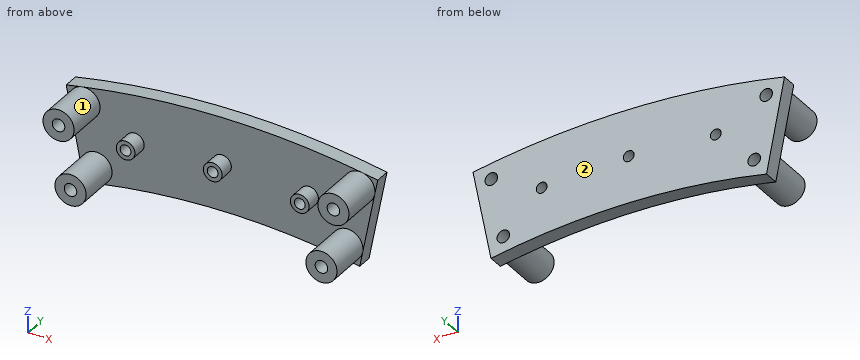
from build123d import *

# Parameters (mm, degrees)
F1_DEPTH = 6.35
F2_R     = 6.35
F3_DEPTH = 17.78
F5_D     = 5.1054
F6_R     = 3.81
F7_DEPTH = 6.35
F9_D     = 4.4


# Not quite as in the source:
# - a pattern or mirror of a feature is missing from the dataset's text; its kind, count and spacing are read off the source's solid


with BuildPart() as f1:
    # F0 (on Front) → F1 (new body)
    with BuildSketch(Plane.XZ):
        with BuildLine():
            Line((56.1730769231, 286.6478596274), (63.5, 324.0367108832))
            ThreePointArc((63.5, 324.0367108832), (0, 330.2), (-63.5, 324.0367108832))
            Line((-63.5, 324.0367108832), (-56.1730769231, 286.6478596274))
            ThreePointArc((-56.1730769231, 286.6478596274), (0, 292.1), (56.1730769231, 286.6478596274))
        make_face()
    extrude(amount=F1_DEPTH)

    # F2 (on face) → F3 (join)
    with BuildSketch(Plane.XZ.offset(6.35)):
        with Locations((-51.149763091, 294.0341888892)):
            Circle(F2_R)
        with Locations((-56.0353976971, 318.9652907527)):
            Circle(F2_R)
    f3 = extrude(amount=F3_DEPTH)

    # F3_copies: F3 across plane
    add(f3.mirror(Plane(origin=(0, 0, 0), x_dir=(0, 0, 1), z_dir=(1, 0, 0))))

    # F5 (through all)
    with Locations(Plane.XZ.offset(24.13)):
        with Locations((-56.0353976971, 318.9652907527), (-51.149763091, 294.0341888892)):
            f5 = Hole(F5_D / 2)

    # F5_copies: F5 across plane
    add(f5.mirror(Plane(origin=(0, 0, 0), x_dir=(0, 0, 1), z_dir=(1, 0, 0))), mode=Mode.SUBTRACT)

    # F6 (on face) → F7 (join)
    with BuildSketch(Plane.XZ.offset(6.35)):
        with Locations((0, 311.15)):
            Circle(F6_R)
        with Locations((-35.501895386, 309.118)):
            Circle(F6_R)
        with Locations((35.501895386, 309.118)):
            Circle(F6_R)
    extrude(amount=F7_DEPTH)

    # F9 (through all)
    with Locations(Plane.XZ.offset(12.7)):
        with Locations((-35.501895386, 309.118), (0, 311.15), (35.501895386, 309.118)):
            Hole(F9_D / 2)


solid = f1.part
Verification items for the finished model (mm, model axes). Face numbers are marked on the shaded views. Give positions to 0.01 mm unless a question says otherwise; leave off trailing zeros. Order: outer loops, then holes, each group sorted by start corner. A loop starts at its lowest first (then second) coordinate and runs counter-clockwise, first axis right, second up. Notation, with made-up numbers: (72.5, 70) -> (93.5, 70) arc R21 ccw to (93.5, 97) -> close; hole circle Ø3 at (69, 8). An arc over 180 degrees is marked (long way). Answer as CSV lines item,"result".
Q1. Depth check by flat-ended pin: pin 1 (6 mm diameter, centred on x = -50, y = -10.5, fed in from +Z); pin 2 (4 mm diameter, centred on x = -1.5, z = 310.5, fed in from -Y); pin 3 (12 mm diameter, centred on x = 50.5, y = -17, fed in from -Z). Enter the tip coordinate at first touch or a pass-through.
Solutions:
pin 1,"stops at z = 324.54"
pin 2,"stops at y = -12.7"
pin 3,"stops at z = 287.68"
Q2. Sectioned sample at A-A on x = 0. Record the cut outline in (y, z), plus the area to 3 significant figures.
Solutions:
outline,"(-12.7, 307.34) -> (-6.35, 307.34) -> (-6.35, 292.1) -> (0, 292.1) -> (0, 308.95) -> (-12.7, 308.95) -> close; (-12.7, 313.35) -> (0, 313.35) -> (0, 330.2) -> (-6.35, 330.2) -> (-6.35, 314.96) -> (-12.7, 314.96) -> close"
area,"234 mm²"
Q3. Scan lines: probe 1 along Z at (x, y) = (0, -8.75); probe 2 along X at (y, z) = (-13.5, 292); probe 3 along X at (y, z) = (-16, 319.5). Record each from-to range of solid material in increasing order.
Solutions:
probe 1,"z = 307.34 to 308.95, 313.35 to 314.96"
probe 2,"x = -57.17 to -52.69, -49.61 to -45.13, 45.13 to 49.61, 52.69 to 57.17"
probe 3,"x = -62.36 to -58.53, -53.54 to -49.71, 49.71 to 53.54, 58.53 to 62.36"
Q4. Sectioned sample at C-C on x = 55. Record the cut outline in (y, z).
Solutions:
outline,"(-24.13, 288.98) -> (-6.35, 288.98) -> (-6.35, 286.88) -> (0, 286.88) -> (0, 316.63) -> (-24.13, 316.63) -> (-24.13, 312.7) -> (-6.35, 312.7) -> (-6.35, 299.08) -> (-24.13, 299.08) -> close; (-24.13, 321.3) -> (0, 321.3) -> (0, 325.59) -> (-6.35, 325.59) -> (-6.35, 325.23) -> (-24.13, 325.23) -> close"
Q5. Sectioned sample at B-B on y = -11.25. Count the separate pieces of the cut face and the enclosed holes in it, plus the area to 3 significant figures.
Solutions:
separate pieces,"7"
enclosed holes,"7"
area,"516 mm²"
Q6. Release check for a two-part mould opening along Z. For the marked faces 1 and 2 record: +Z half, -Z half, draft (parallel to the pull), parting line (faces both ways), or undercut.
Solutions:
face 1,"undercut"
face 2,"draft"
Q7. Sectioned sample at D-D on x = -23. Record the cut outline in (y, z).
Solutions:
outline,"(-6.35, 291.19) -> (0, 291.19) -> (0, 329.4) -> (-6.35, 329.4) -> close"
